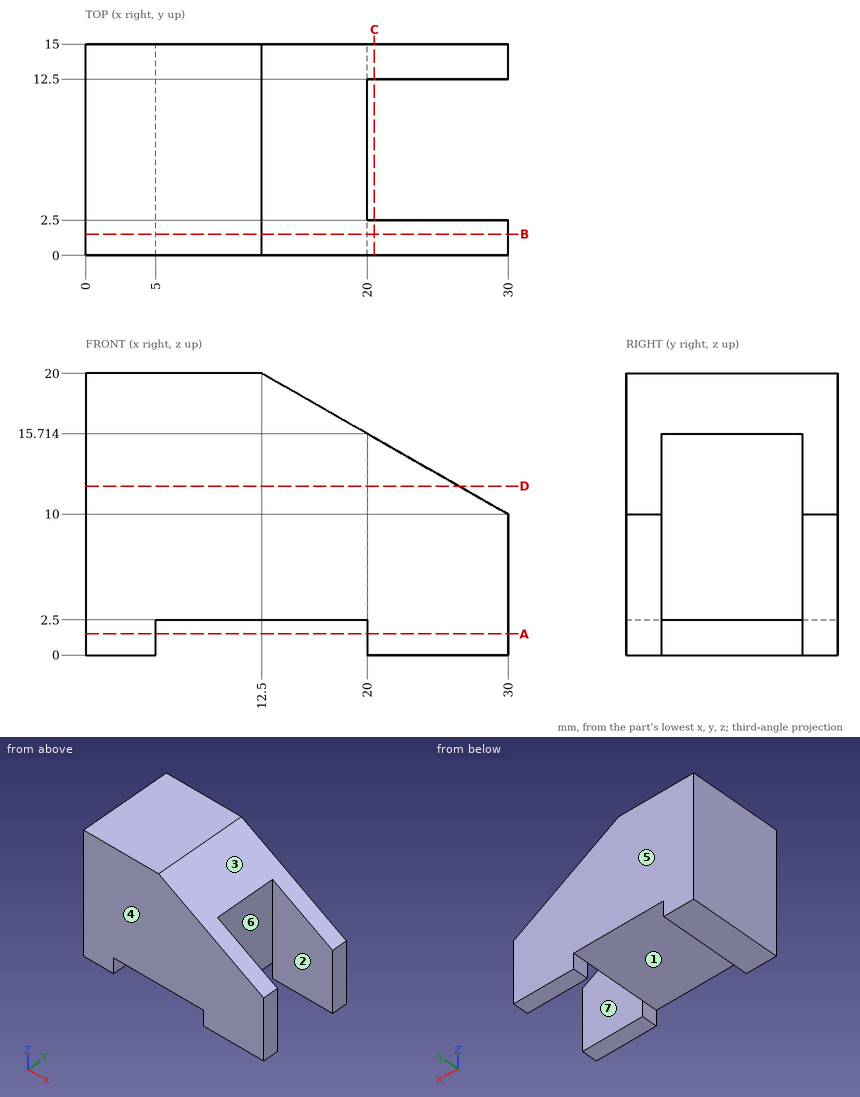
The drawing under review shows one solid part. Ordinate dimensions are in mm from its lowest x, y, z. A direction names the side the tool comes from. Give positions to 0.01 mm unless a question says otherwise; leave off trailing zeros. Loops run counter-clockwise (first coordinate to the right, second up) from the corner with the lowest first, then second, coordinate; pieces in that order, holes last. Notation, with made-up numbers: M 19,42.25 L 55,42.25 A24 cw 55,73.25 Z; hole C 41,65.5 d7. An arc over 180 degrees is marked long. Return JSON: item names as keys, results as strings. Group by question number.
Item 1: We need section B-B (y = 1.5). Give the boundary of the cut face in (x, z), and give its area (3 significant figures).
Item 2: We need section D-D (z = 12). Give the boundary of the cut face in (x, y).
Item 3: We need section C-C (x = 20.5). Give the boundary of the cut face in (y, z).
Item 4: For probe 1 along Y at (x, z) = (24.5, 10.5); probe 2 along X at (y, z) = (1.75, 1.5); probe 3 along X at (y, z) = (6.75, 1.5), list the stretches that pass through material, from the lowest coordinate up.
Item 5: Insertion check: pin 1 Ø1.5 at (y, z) = (8, 12.5) entering from +X; pin 2 Ø7.5 at (x, y) = (9, 4) entering from -Z. Each pin has a flat end and moves straight along its axis. Give the tip position at first contact, or say it passes through.
Item 6: We need section A-A (z = 1.5). Give the boundary of the cut face in (x, y), and give its area (3 significant figures).
Item 7: Mouldability with a two-part tool opening along Y and no side actions: class the marked faces 4, 5, 6 and 7 as released by +Y, released by -Y, zero draft, split by the parting line, or undercut.
Item 8: Tool access review of the marked faces 1, 2 and 3: name each direction out of +Z, -Z, +X, -X, +Y, -Y from which nothing blocks a thin tool from reaching the whole face with its end or side.
Output:
{
 "1": {"outline": "M 0,0 L 5,0 L 5,2.5 L 20,2.5 L 20,0 L 30,0 L 30,10 L 12.5,20 L 0,20 Z", "area": "475 mm^2"},
 "2": {"outline": "M 0,0 L 26.5,0 L 26.5,2.5 L 20,2.5 L 20,12.5 L 26.5,12.5 L 26.5,15 L 0,15 Z"},
 "3": {"outline": "M 0,0 L 2.5,0 L 2.5,15.43 L 0,15.43 Z; M 12.5,0 L 15,0 L 15,15.43 L 12.5,15.43 Z"},
 "4": {"probe 1": "y = 0 to 2.5, 12.5 to 15", "probe 2": "x = 0 to 5, 20 to 30", "probe 3": "x = 0 to 5"},
 "5": {"pin 1": "stops at x = 20", "pin 2": "stops at z = 2.5"},
 "6": {"outline": "M 0,0 L 5,0 L 5,15 L 0,15 Z; M 20,0 L 30,0 L 30,2.5 L 20,2.5 Z; M 20,12.5 L 30,12.5 L 30,15 L 20,15 Z", "area": "125 mm^2"},
 "7": {"face 4": "released by -Y", "face 5": "released by +Y", "face 6": "undercut", "face 7": "undercut"},
 "8": {"face 1": "-Z, +Y, -Y", "face 2": "+Z, -Z, +X", "face 3": "+Z, +X, +Y, -Y"}
}
